Verification items for the finished model (mm, model axes). Give positions to 0.01 mm unless a question says otherwise; leave off trailing zeros. Loops run counter-clockwise (first coordinate to the right, second up) from the corner with the lowest first, then second, coordinate; pieces in that order, holes last. Notation, with made-up numbers: (-8.75, -34.75) - (48.25, -34.75) arc R26 ccw to (48.25, 2.25) - close; hole circle Ø3 at (4.5, 27.25). An arc over 180 degrees is marked (long way). One line per item, written item: value. Start each with the question number.
1. Scan lines: L1, parallel to X at y = 11, z = 0.4; L2, parallel to Y at x = -1, z = -0.2; L3, parallel to X at y = -3, z = -0.65. Record each from-to range of solid material in increasing order. Write a range as [from, to].
2. Gauge pin test, flat ends, axial feed: pin 1 (1.5 mm diameter, centred on x = -0.5, y = -6.5, fed in from +Z); pin 2 (5.5 mm diameter, centred on x = 40, y = -1, fed in from +Z); pin 3 (1.5 mm diameter, centred on x = -37, z = 0, fed in from +Y); pin 4 (2 mm diameter, centred on y = 3.5, z = -1, fed in from +X). Record the tip position at first contact, or that the pin passes through.
3. Sectioned sample at C-C (x = -21). Record the cut outline in (y, z), plus the area to 3 significant figures.
4. Sectioned sample at B-B (y = 1). Count the separate pieces of the cut face and the enclosed holes in it, plus the area to 3 significant figures.
5. Sectioned sample at A-A (x = 0). Record the cut outline in (y, z), plus the area to 4 significant figures.
from build123d import *

# Parameters (mm, degrees)
BOSS_EXTRUDE2_DEPTH      = 2.5
SKETCH3_R                = 4.5
CUT_EXTRUDE3_DEPTH       = 8
SKETCH4_R                = 5
CUT_EXTRUDE4_DEPTH       = 1.5
SKETCH5_R                = 3.25
CUT_EXTRUDE5_DEPTH       = 10
CHAMFER6_SIZE            = 1
CHAMFER6_OF_MIRROR7_SIZE = 1
SKETCH6_R                = 2
CUT_EXTRUDE6_DEPTH       = 3
SKETCH7_R                = 1.5
CUT_EXTRUDE7_DEPTH       = 3
SKETCH8_R                = 1.5
CUT_EXTRUDE8_DEPTH       = 3


with BuildPart() as part:
    # Sketch1 → Boss-Extrude2 (new body, symmetric)
    with BuildSketch(Plane.XY):
        with BuildLine():
            Line((-44.599094606, 4.924384255), (-20.111639684, 23.933975293))
            ThreePointArc((-20.111639684, 23.933975293), (-18.64459039, 24.726101678), (-17, 25))
            Line((-17, 25), (17, 25))
            ThreePointArc((17, 25), (18.64459039, 24.726101678), (20.111639684, 23.933975293))
            Line((20.111639684, 23.933975293), (44.599094606, 4.924384255))
            ThreePointArc((44.599094606, 4.924384255), (47.095170256, -3.430752773), (40, -8.5))
            Line((40, -8.5), (-40, -8.5))
            ThreePointArc((-40, -8.5), (-47.095170256, -3.430752773), (-44.599094606, 4.924384255))
        make_face()
    extrude(amount=BOSS_EXTRUDE2_DEPTH, both=True)

    # Sketch3 → Cut-Extrude3 (cut)
    with BuildSketch(Plane(origin=(0, 0, -2.5), x_dir=(-1, 0, 0), z_dir=(0, 0, -1))):
        with Locations((-40, -1)):
            Circle(SKETCH3_R)
    cut_extrude3 = extrude(amount=-CUT_EXTRUDE3_DEPTH, mode=Mode.SUBTRACT)

    # Sketch4 → Cut-Extrude4 (cut)
    with BuildSketch(Plane(origin=(0, 0, -2.5), x_dir=(-1, 0, 0), z_dir=(0, 0, -1))):
        with Locations((-40, -1)):
            Circle(SKETCH4_R)
    cut_extrude4 = extrude(amount=-CUT_EXTRUDE4_DEPTH, mode=Mode.SUBTRACT)

    # Mirror1: Cut-Extrude3, Cut-Extrude4 across plane
    add(cut_extrude3.mirror(Plane(origin=(0, 0, 0), x_dir=(0, 0, 1), z_dir=(1, 0, 0))), mode=Mode.SUBTRACT)
    add(cut_extrude4.mirror(Plane(origin=(0, 0, 0), x_dir=(0, 0, 1), z_dir=(1, 0, 0))), mode=Mode.SUBTRACT)

    # Sketch5 → Cut-Extrude5 (cut)
    with BuildSketch(Plane(origin=(0, 0, -2.5), x_dir=(-1, 0, 0), z_dir=(0, 0, -1))):
        with Locations((-15, 0)):
            Circle(SKETCH5_R)
    cut_extrude5 = extrude(amount=-CUT_EXTRUDE5_DEPTH, mode=Mode.SUBTRACT)

    # Chamfer6
    chamfer6_edges = [part.edges().sort_by_distance(p)[0] for p in [
        (18.25, 0, 2.5),
        (18.25, 0, -2.5),
    ]]
    chamfer(chamfer6_edges, length=CHAMFER6_SIZE)

    # Mirror7: Cut-Extrude5 across plane
    add(cut_extrude5.mirror(Plane(origin=(0, 0, 0), x_dir=(0, 0, 1), z_dir=(1, 0, 0))), mode=Mode.SUBTRACT)

    # Chamfer6 of Mirror7
    chamfer6_of_mirror7_edges = [part.edges().sort_by_distance(p)[0] for p in [
        (-18.25, 0, 2.5),
        (-18.25, 0, -2.5),
    ]]
    chamfer(chamfer6_of_mirror7_edges, length=CHAMFER6_OF_MIRROR7_SIZE)

    # Sketch6 → Cut-Extrude6 (cut)
    with BuildSketch(Plane(origin=(0, 0, -2.5), x_dir=(-1, 0, 0), z_dir=(0, 0, -1))):
        with Locations((0, 15)):
            Circle(SKETCH6_R)
        with Locations((30, 12.5)):
            Circle(SKETCH6_R)
        with Locations((-30, 12.5)):
            Circle(SKETCH6_R)
    extrude(amount=-CUT_EXTRUDE6_DEPTH, mode=Mode.SUBTRACT)

    # Sketch7 → Cut-Extrude7 (cut)
    with BuildSketch(Plane.XY.offset(2.5)):
        with Locations((21, 20.079456047)):
            Circle(SKETCH7_R)
        with Locations((0, -6)):
            Circle(SKETCH7_R)
        with Locations((-21, 20.079456047)):
            Circle(SKETCH7_R)
    extrude(amount=-CUT_EXTRUDE7_DEPTH, mode=Mode.SUBTRACT)

    # Sketch8 → Cut-Extrude8 (cut)
    with BuildSketch(Plane.XY.offset(2.5)):
        with Locations((0, 22.5)):
            Circle(SKETCH8_R)
    extrude(amount=-CUT_EXTRUDE8_DEPTH, mode=Mode.SUBTRACT)


solid = part.part
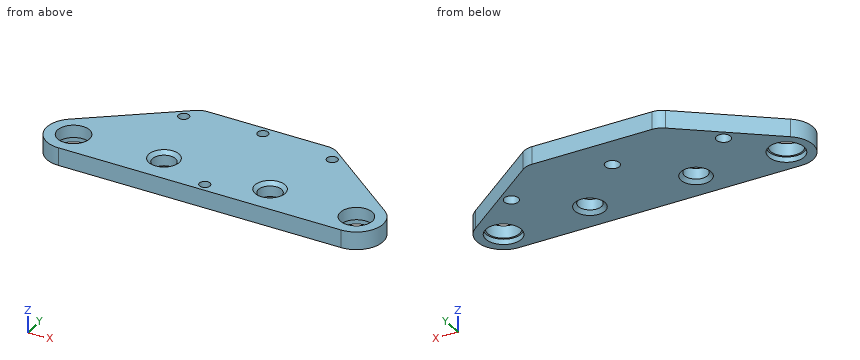
Results are:
1. L1: x = [-36.77, -31.32], [-28.68, 28.68], [31.32, 36.77]
1. L2: y = [-8.5, -7.12], [-4.88, 13.27], [16.73, 21.38], [23.62, 25]
1. L3: x = [-47.23, -44.03], [-35.97, -16.25], [-13.75, 13.75], [16.25, 35.97], [44.03, 47.23]
2. pin 1: stops at z = -0.5
2. pin 2: passes through
2. pin 3: stops at y = 11.41
2. pin 4: stops at x = 46.63
3. outline: (-8.5, -2.5) - (23.24, -2.5) - (23.24, 2.5) - (21.58, 2.5) - (21.58, -0.5) - (18.58, -0.5) - (18.58, 2.5) - (-8.5, 2.5) - close
3. area: 150 mm^2
4. separate pieces: 5
4. enclosed holes: 0
4. area: 322 mm^2
5. outline: (-8.5, -2.5) - (13, -2.5) - (13, 0.5) - (17, 0.5) - (17, -2.5) - (25, -2.5) - (25, 2.5) - (24, 2.5) - (24, -0.5) - (21, -0.5) - (21, 2.5) - (-4.5, 2.5) - (-4.5, -0.5) - (-7.5, -0.5) - (-7.5, 2.5) - (-8.5, 2.5) - close
5. area: 137.5 mm^2
